Could you check a few things on this drawing? It's one solid part, dimensions in mm from its lowest x, y, z. Round coordinates to 2 decimals unless told otherwise and drop trailing zeros. Write each loop counter-clockwise with the first axis right and the second up, starting at its lowest first coordinate (ties: lowest second). Pieces come first, ordered by that corner, then holes. Notation, with made-up numbers: M 1.5,27 L 22.5,27 A34 ccw 22.5,58 Z; hole C -4,-17 d7. An arc over 180 degrees is marked long. One line per item, written item: value. Start each with the question number.
(1) I want a section at C-C on x = 14.75. Please give me the cut outline in (y, z).
(2) I want a section at D-D on y = 0.8. Count the separate pieces of the cut face and the enclosed holes in it.
(3) I want a section at A-A on z = 10. Please give me the cut outline in (x, y).
(4) I want a section at B-B on z = 17.5. Please give me the cut outline in (x, y).
(5) If I drill on L1, parallel to Z at x = 9.5, y = 0.1 (1 decimal); L2, parallel to X at y = 0.85, z = 3, over which ranges is the centre line in solid material (lowest first)?
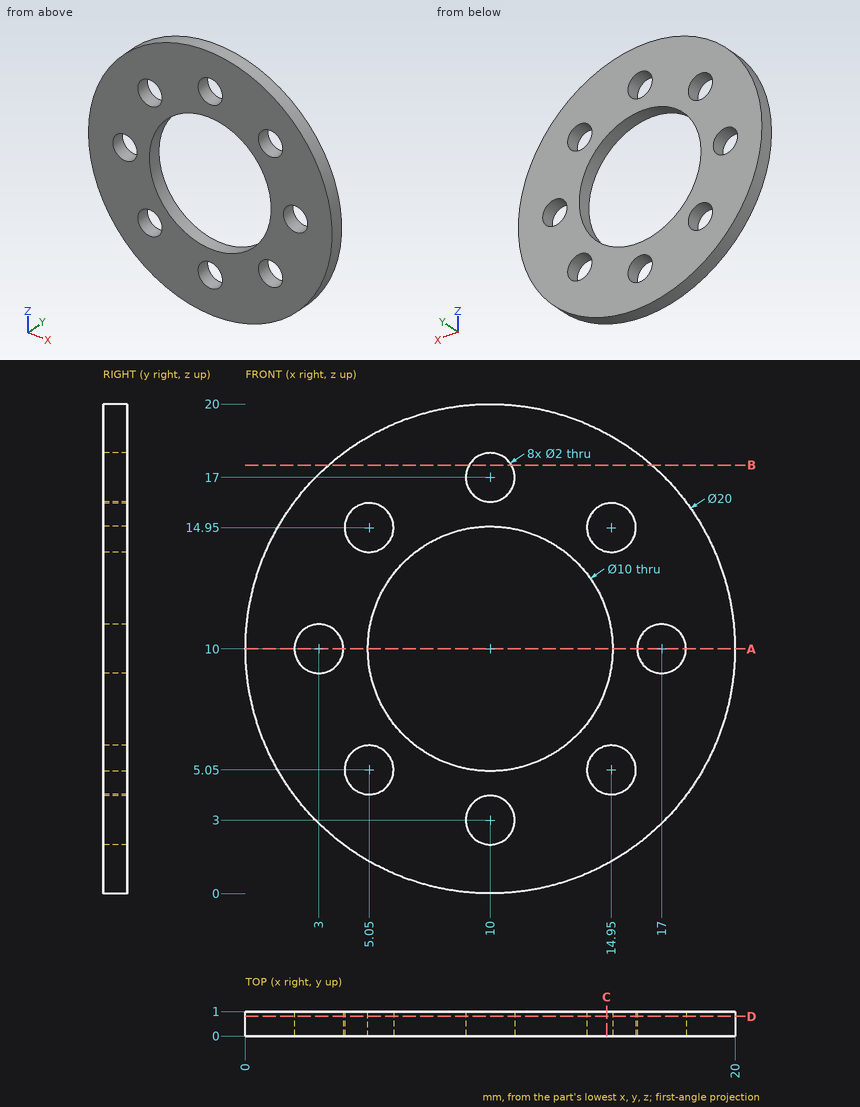
Found:
1. outline: M 0,1.2 L 1,1.2 L 1,4.07 L 0,4.07 Z; M 0,6.03 L 1,6.03 L 1,8.44 L 0,8.44 Z; M 0,11.56 L 1,11.56 L 1,13.97 L 0,13.97 Z; M 0,15.93 L 1,15.93 L 1,18.8 L 0,18.8 Z
2. separate pieces: 1
2. enclosed holes: 9
3. outline: M 0,0 L 2,0 L 2,1 L 0,1 Z; M 4,0 L 5,0 L 5,1 L 4,1 Z; M 15,0 L 16,0 L 16,1 L 15,1 Z; M 18,0 L 20,0 L 20,1 L 18,1 Z
4. outline: M 3.39,0 L 9.13,0 L 9.13,1 L 3.39,1 Z; M 10.87,0 L 16.61,0 L 16.61,1 L 10.87,1 Z
5. L1: z = 0 to 2.1, 3.9 to 5, 15 to 16.1, 17.9 to 20
5. L2: x = 2.86 to 9, 11 to 17.14
